```python
from build123d import *

# Parameters (mm, degrees)
F0_W     = 30
F0_H     = 30
F0_R     = 10
F1_DEPTH = 15
F1_TAPER = -3
F2_DEPTH = 10
F3_R     = 2


with BuildPart() as f1:
    # F0 (on Top) → F1 (new body)
    with BuildSketch(Plane.XY):
        with Locations((-58.3209823817, -55.5250146758)):
            Rectangle(F0_W, F0_H)
        with Locations((-58.3209823817, -55.5250146758)):
            Circle(F0_R, mode=Mode.SUBTRACT)
    extrude(amount=F1_DEPTH, taper=F1_TAPER)

    # F0 (on Top) → F2 (join)
    with BuildSketch(Plane.XY):
        with Locations((-58.3209823817, -55.5250146758)):
            Circle(F0_R)
    extrude(amount=F2_DEPTH)

    # F3
    f3_edges = [f1.edges().sort_by_distance(p)[0] for p in [
        (-67.796905, -55.525015, 10),
        (-67.534866, -55.525015, 15),
        (-42.534866, -55.525015, 15),
        (-58.320982, -39.738898, 15),
        (-58.320982, -71.311131, 15),
        (-74.107099, -55.525015, 15),
        (-58.320982, -40.525015, 0),
        (-73.320982, -55.525015, 0),
        (-58.320982, -70.525015, 0),
        (-43.320982, -55.525015, 0),
        (-42.927924, -70.918073, 7.5),
        (-42.927924, -40.131956, 7.5),
        (-73.714041, -70.918073, 7.5),
        (-73.714041, -40.131956, 7.5),
    ]]
    fillet(f3_edges, radius=F3_R)


solid = f1.part
```
Design review of the part built by this model. Coordinates are the model's own, in mm. Give positions to 0.01 mm unless a question says otherwise; leave off trailing zeros.
(1) Mouldability with a two-part tool opening along Y and no side actions: class faces 1 (the face through (-58, -55, 10)), 2 (the face through (-59, -55, 0)) as +Y half, -Y half, draft (parallel to the pull), parting line (faces both ways), or undercut.
Checked values:
face 1: undercut
face 2: draft
(2) Clearance check with flat-ended pins moving along their axes: pin 1 Ø1.5 at (x, z) = (-50.5, 8) entering from +Y; pin 2 Ø12 at (x, y) = (-55.5, -54.5) entering from +Z; pin 3 Ø1.5 at (y, z) = (-67, 3.5) entering from -X. State where each tip first meets the part, or that it passes through.
Checked values:
pin 1: stops at y = -40.07
pin 2: stops at z = 10.85
pin 3: stops at x = -73.54
(3) Wall thickness on line 1 along Z through (x, y) = (-61.5, -57.5); line 2 along X through (y, z) = (-62, 13.75); line 3 along Y through (x, z) = (-51, 2.5): over which ranges is each line inside the solid? List them lowest first.
Checked values:
line 1: z = 0 to 10
line 2: x = -73.85 to -65.23, -51.41 to -42.79
line 3: y = -70.66 to -40.39
